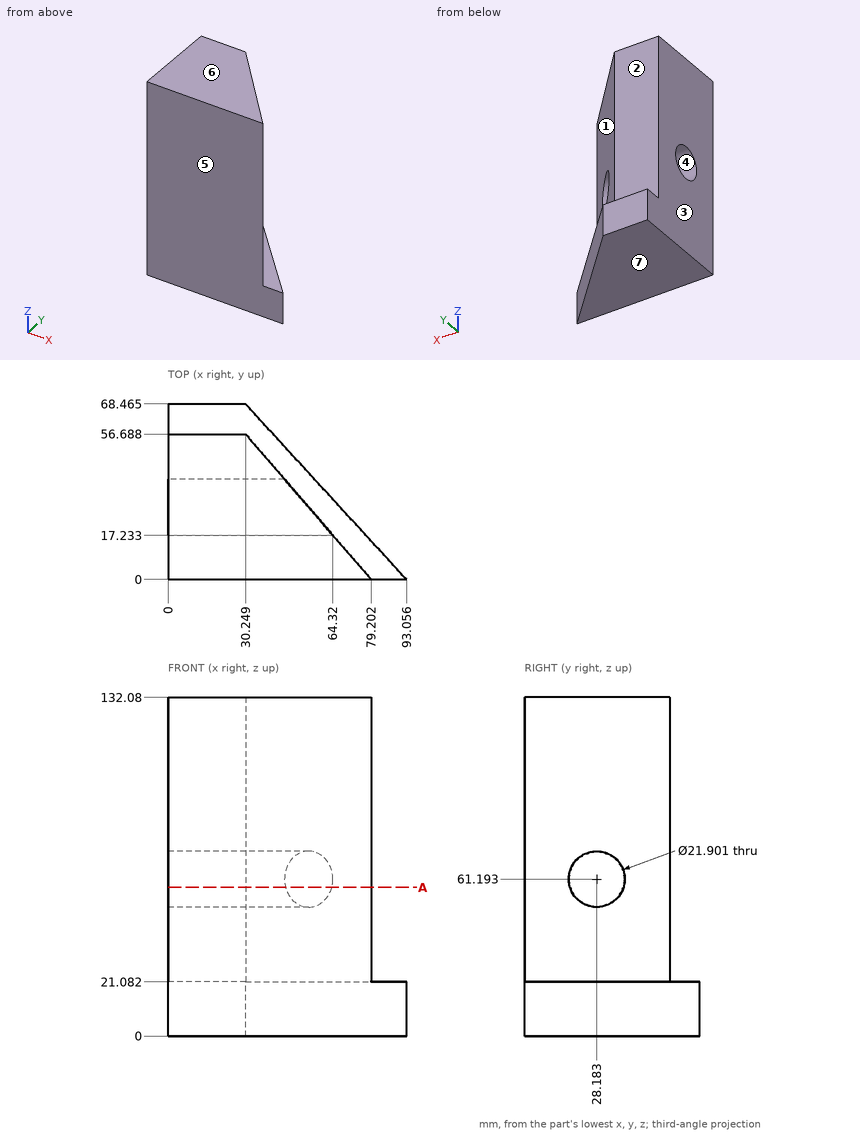
Part print with two shaded views. Sizes in mm from the minimum x, y, z corner. A direction names the side the tool comes from. Round coordinates to 2 decimals unless told otherwise and drop trailing zeros. Order: outer loops, then holes, each group sorted by start corner. A loop starts at its lowest first (then second) coordinate and runs counter-clockwise, first axis right, second up. Notation, with made-up numbers: M 77,-2.75 L 82,-2.75 A22 cw 82,33.25 Z; hole C 58,-11.5 d5. An arc over 180 degrees is marked long. Answer in a Markdown table with one row per item. Add a question column.
Q1. Pin check, flat tips, straight feed: pin 1 (9 mm diameter, centred on x = 10.5, z = 98, fed in from +Y); pin 2 (17.5 mm diameter, centred on y = 28.18, z = 61.19, fed in from -X); pin 3 (3 mm diameter, centred on x = 80.5, z = 86, fed in from +Y) (1 decimal). Stop position of each tip, or through.
Q2. Mould opens along Z. For the marked faces 4, 5, 6 and 7 say: +Z half, -Z half, draft (parallel to the pull), parting line (faces both ways), or undercut.
Q3. Cut at A-A on z = 58. Give the cut face in (x, y).
Q4. Wall check: L1, parallel to Z at x = 42.5, y = 28; L2, parallel to Y at x = 19, z = 116; L3, parallel to Z at x = 47, y = 43. Give the ranges that are in metal, low to high. Write a range as from..to.
Q5. 3-axis set-ups, long thin cutter, end or side, ignore diameter. For the marked faces 1, 2 and 3: which of +Z, -Z, +X, -X, +Y, -Y reach the whole face in a straight line?
Established:
| question | item | result |
|---|---|---|
| 1 | pin 1 | stops at y = 56.69 |
| 1 | pin 2 | passes through |
| 1 | pin 3 | stops at y = 0.2 |
| 2 | face 4 | undercut |
| 2 | face 5 | draft |
| 2 | face 6 | +Z half |
| 2 | face 7 | -Z half |
| 3 | outline | M 0,0 L 79.2,0 L 63.91,17.71 L 0,17.71 Z; M 0,38.66 L 45.82,38.66 L 30.25,56.69 L 0,56.69 Z |
| 4 | L1 | z = 0..50.24, 72.14..132.08 |
| 4 | L2 | y = 0..56.69 |
| 4 | L3 | z = 0..21.08 |
| 5 | face 1 | +Z, +X, +Y |
| 5 | face 2 | +Z, +X, -X, +Y |
| 5 | face 3 | +Z, -Z, -X, +Y, -Y |
